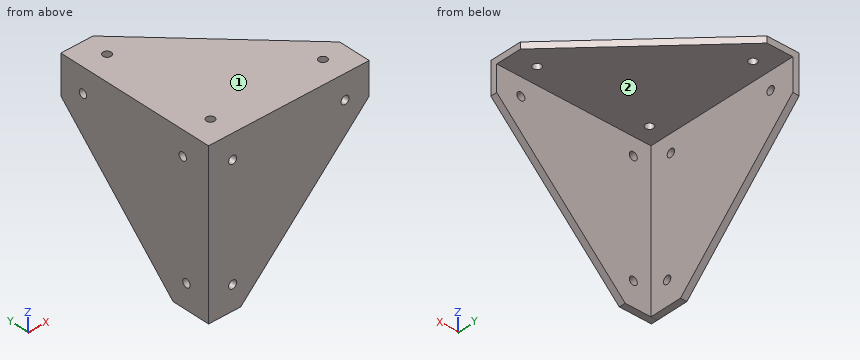
```python
from build123d import *

# Parameters (mm, degrees)
F1_DEPTH  = 4
F4_DEPTH  = 4
F9_DEPTH  = 4
F10_R     = 2
F11_DEPTH = 4
F12_R     = 2.5
F13_DEPTH = 4
F14_R     = 2.5
F15_DEPTH = 4
F16_R     = 2.5
F17_DEPTH = 4


with BuildPart() as f1:
    # F0 (on Top) → F1 (new body)
    with BuildSketch(Plane.XY):
        Polygon((-28.663731938, 61.6347389425), (-48.663731938, 61.6347389425), (-48.663731938, -38.3652610575), (51.336268062, -38.3652610575), (51.336268062, -18.3652610575), align=None)
    extrude(amount=F1_DEPTH)



with BuildPart() as f4:
    # F3 (on offset) → F4 (new body)
    with BuildSketch(Plane(origin=(-48.663731938, 0, 0), x_dir=(0, -1, 0), z_dir=(-1, 0, 0))):
        Polygon((38.3652610575, 0), (-61.6347389425, 0), (-61.6347389425, -20), (14.3654177458, -95.9132762154), (38.3652610575, -96), align=None)
    extrude(amount=-F4_DEPTH)


with BuildPart() as f1_1:
    add(f1.part)

    add(f4.part)  # F9 merges F4
    # F8 (on offset) → F9 (join)
    with BuildSketch(Plane.XZ.offset(38.3652610575)):
        Polygon((51.336268062, -16), (51.336268062, 4), (-48.663731938, 4), (-48.663731938, -96), (-28.663731938, -96), align=None)
    extrude(amount=-F9_DEPTH)

    # F10 (on face) → F11 (cut)
    with BuildSketch(Plane.XZ.offset(38.3652610575)):
        with Locations((36.336268062, -11)):
            Circle(F10_R)
        with Locations((-33.663731938, -11)):
            Circle(F10_R)
        with Locations((-33.663731938, -81)):
            Circle(F10_R)
    extrude(amount=-F11_DEPTH, mode=Mode.SUBTRACT)

    # F12 (on face) → F13 (cut)
    with BuildSketch(Plane.XZ.offset(38.3652610575)):
        with Locations((36.336268062, -11)):
            Circle(F12_R)
        with Locations((-33.663731938, -11)):
            Circle(F12_R)
        with Locations((-33.663731938, -81)):
            Circle(F12_R)
    extrude(amount=-F13_DEPTH, mode=Mode.SUBTRACT)

    # F14 (on face) → F15 (cut)
    with BuildSketch(Plane(origin=(-48.663731938, 0, 0), x_dir=(0, -1, 0), z_dir=(-1, 0, 0))):
        with Locations((-46.6681093954, -11)):
            Circle(F14_R)
        with Locations((20.8652610575, -11)):
            Circle(F14_R)
        with Locations((23.3652610575, -80.9456993499)):
            Circle(F14_R)
    extrude(amount=-F15_DEPTH, mode=Mode.SUBTRACT)

    # F16 (on face) → F17 (cut)
    with BuildSketch(Plane.XY.offset(4)):
        with Locations((-33.663731938, 46.6347389425)):
            Circle(F16_R)
        with Locations((-33.663731938, -23.3652610575)):
            Circle(F16_R)
        with Locations((36.336268062, -23.3652610575)):
            Circle(F16_R)
    extrude(amount=-F17_DEPTH, mode=Mode.SUBTRACT)


solid = f1_1.part
```
The listing builds one solid part. Answer for the finished solid, in the listing's coordinates (mm). Face numbers are marked on the shaded views. A direction names the side the tool comes from. Give positions to 0.01 mm unless a question says otherwise; leave off trailing zeros. Write each loop counter-clockwise with the first axis right and the second up, starting at its lowest first coordinate (ties: lowest second). Pieces come first, ordered by that corner, then holes. Notation, with made-up numbers: (-7, -14.75) -> (21, -14.75) arc R23 cw to (21, 2.25) -> close; hole circle Ø7 at (-24, 70.5). An arc over 180 degrees is marked (long way). Use one line per item in the form item = value.
1) Section A-A on z = -11 is taken. Write down the section's boundary in (x, y), plus the area to 3 significant figures.
Result:
outline = (-48.66, -38.37) -> (-36.16, -38.37) -> (-36.16, -34.37) -> (-44.66, -34.37) -> (-44.66, -23.37) -> (-48.66, -23.37) -> close; (-48.66, -18.37) -> (-44.66, -18.37) -> (-44.66, 44.17) -> (-48.66, 44.17) -> close; (-48.66, 49.17) -> (-44.66, 49.17) -> (-44.66, 61.63) -> (-48.66, 61.63) -> close; (-31.16, -38.37) -> (33.84, -38.37) -> (33.84, -34.37) -> (-31.16, -34.37) -> close; (38.84, -38.37) -> (51.34, -38.37) -> (51.34, -34.37) -> (38.84, -34.37) -> close
area = 704 mm²
2) Each of these flat-tipped pins is pushed along its axis until it touches: P1, Ø6, axis at x = 36.34, y = -23.37, coming from the -Z side; P2, Ø6, axis at y = -20.87, z = -11, coming from the -X side; P3, Ø2, axis at x = -7.5, z = -70, coming from the +Y side; P4, Ø2, axis at y = 15.5, z = -10, coming from the +X side. Where does it stop, or does it pass through?
Result:
P1 = 0
P2 = -48.66
P3 = -34.37
P4 = -44.66
3) Section C-C on y = 23 is taken. Write down the section's boundary in (x, z), plus the area to 3 significant figures.
Result:
outline = (-48.66, -58.59) -> (-44.66, -58.59) -> (-44.66, 0) -> (9.97, 0) -> (9.97, 4) -> (-48.66, 4) -> close
area = 469 mm²
4) Section B-B on x = -38 is taken. Write down the section's boundary in (y, z).
Result:
outline = (-38.37, -96) -> (-34.37, -96) -> (-34.37, 0) -> (61.63, 0) -> (61.63, 4) -> (-38.37, 4) -> close
5) Straight lines are drawn through the part: probe 1 along X at (y, z) = (-6, -20); probe 2 along Z at (x, y) = (27, -10); probe 3 along Y at (x, z) = (24, -35.5). For each, find the intervals that lie inside material, in ascending order.
Result:
probe_1 = -48.66 to -44.66
probe_2 = 0 to 4
probe_3 = -38.37 to -34.37
6) A tool of negligible diameter and unlimited length cuts with its end or side. For the marked faces 1 and 2, from which of +Z, -Z, +X, -X, +Y, -Y can it reach the whole face along a straight path? Write none if from no direction.
Result:
face_1 = +Z, +X, -X, +Y, -Y
face_2 = -Z, +X, +Y
